from build123d import *

# Parameters (mm, degrees)
F0_W     = 19.05
F0_H     = 9.525
F1_DEPTH = 4.699
F2_R     = 2.54
F3_DEPTH = 4.699
F4_R     = 1.190625
F5_DEPTH = 9.399
F6_W     = 3.5052
F6_H     = 9.525
F7_DEPTH = 19.051


with BuildPart() as f1:
    # F0 (on Right) → F1 (new body, symmetric)
    with BuildSketch(Plane.YZ):
        with Locations((0, 4.7625)):
            Rectangle(F0_W, F0_H)
    extrude(amount=F1_DEPTH, both=True)

    # F2 (on Right) → F3 (join, symmetric)
    with BuildSketch(Plane.YZ):
        with BuildLine():
            ThreePointArc((-9.525, 17.4625), (-3.175, 11.1125), (3.175, 17.4625))
            ThreePointArc((3.175, 17.4625), (-3.175, 23.8125), (-9.525, 17.4625))
        make_face()
        with Locations((-3.175, 17.4625)):
            Circle(F2_R, mode=Mode.SUBTRACT)
        with BuildLine():
            Line((3.175, 0), (3.175, 17.4625))
            ThreePointArc((3.175, 17.4625), (-3.175, 11.1125), (-9.525, 17.4625))
            Line((-9.525, 17.4625), (-9.525, 0))
            Line((-9.525, 0), (3.175, 0))
        make_face()
    extrude(amount=F3_DEPTH, both=True)

    # F4 (on face) → F5 (cut, through all)
    with BuildSketch(Plane.YZ.offset(4.699)):
        with Locations((-3.175, 4.7625)):
            Circle(F4_R)
        with Locations((3.175, 4.7625)):
            Circle(F4_R)
    extrude(amount=-F5_DEPTH, mode=Mode.SUBTRACT)

    # F6 (on face) → F7 (cut, through all)
    with BuildSketch(Plane.XZ.offset(9.525)):
        with Locations((0, 23.8125)):
            Rectangle(F6_W, F6_H)
        with Locations((0, 14.2875)):
            Rectangle(F6_W, F6_H)
    extrude(amount=-F7_DEPTH, mode=Mode.SUBTRACT)


solid = f1.part
The listing builds one solid part. Answer for the finished solid, in the listing's coordinates (mm). A direction names the side the tool comes from. Give positions to 0.01 mm unless a question says otherwise; leave off trailing zeros. Loops run counter-clockwise (first coordinate to the right, second up) from the corner with the lowest first, then second, coordinate; pieces in that order, holes last.
Item 1: This flat-tipped pin is pushed along its axis until it touches: pin 1 Ø3 at (x, z) = (4, 13.5) entering from +Y (3 decimals). Where does it stop, or does it pass through?
Derived:
pin 1: stops at y = 3.175
Item 2: A cutting plane is placed at A-A (y = -1). Give the vertices of the cut face in (x, z) (3 decimals), then the cut area to 3 significant figures.
Derived:
outline: (-4.699, 0) - (4.699, 0) - (4.699, 16.151) - (1.753, 16.151) - (1.753, 9.525) - (-1.753, 9.525) - (-1.753, 16.151) - (-4.699, 16.151) - close; (-4.699, 18.774) - (-1.753, 18.774) - (-1.753, 23.428) - (-4.699, 23.428) - close; (1.753, 18.774) - (4.699, 18.774) - (4.699, 23.428) - (1.753, 23.428) - close
area: 156 mm2
Item 3: Find the intervals of material crossed by line 1 along Z through (x, y) = (4.25, -3.25); line 2 along X through (y, z) = (-6.75, 18); line 3 along Z through (x, y) = (-3.5, 7.25) (3 decimals), in increasing order.
Derived:
line 1: z = 0 to 3.57, 5.95 to 14.92, 20 to 23.81
line 2: x = -4.7 to -1.75, 1.75 to 4.7
line 3: z = 0 to 9.525
Item 4: Determine the mould class of faces 1 (the flat face through (1.753, -5, 15)), 2 (the flat face through (0, 9.525, 5)), 3 (the cylindrical face through (0.066, -3.33, 5.943)) for opening direction Y: +Y half, -Y half, draft (parallel to the pull), parting line (faces both ways), or undercut.
Derived:
face 1: draft
face 2: +Y half
face 3: undercut
Item 5: A cutting plane is placed at D-D (y = 2.5). Give the vertices of the cut face in (x, z) (3 decimals).
Derived:
outline: (-4.699, 0) - (4.699, 0) - (4.699, 3.782) - (-4.699, 3.782) - close; (-4.699, 5.743) - (4.699, 5.743) - (4.699, 20.312) - (1.753, 20.312) - (1.753, 9.525) - (-1.753, 9.525) - (-1.753, 20.312) - (-4.699, 20.312) - close
Item 6: A cutting plane is placed at B-B (z = 20.75). Give the vertices of the cut face in (x, y), then the cut area to 3 significant figures.
Derived:
outline: (-4.7, -8.61) - (-1.75, -8.61) - (-1.75, 2.26) - (-4.7, 2.26) - close; (1.75, -8.61) - (4.7, -8.61) - (4.7, 2.26) - (1.75, 2.26) - close
area: 64.0 mm2
Item 7: A cutting plane is placed at C-C (x = 1). Give the vertices of the cut face in (y, z) (1 decimal).
Derived:
outline: (-9.5, 0) - (9.5, 0) - (9.5, 9.5) - (-9.5, 9.5) - close; hole circle Ø2.4 at (-3.2, 4.8); hole circle Ø2.4 at (3.2, 4.8)
Item 8: A tool of negligible diameter and unlimited length cuts with its end or side. For faces 4 (the flat face through (0, 2, 9.525)), 5 (the flat face through (3, 3.175, 13)), 6 (the flat face through (-1.753, -2, 15)), from which of +Z, -Z, +X, -X, +Y, -Y can it reach the whole face along a straight path? Write none if from no direction.
Derived:
face 4: +Z, +Y
face 5: +Z, +X, -X, +Y
face 6: +Z, +Y, -Y
